Work out the finished part from the listing and answer in its coordinate system (mm). Face numbers are marked on the shaded views. A direction names the side the tool comes from. Coordinates: 2 decimals unless noted, no trailing zeros. Loops run counter-clockwise (first coordinate to the right, second up) from the corner with the lowest first, then second, coordinate; pieces in that order, holes last. Notation, with made-up numbers: (42.5, 66) -> (70.5, 66) arc R25 ccw to (70.5, 96) -> close; hole circle Ø6 at (34, 47.25). An arc over 180 degrees is marked (long way). One line per question, with ' | ' between items.
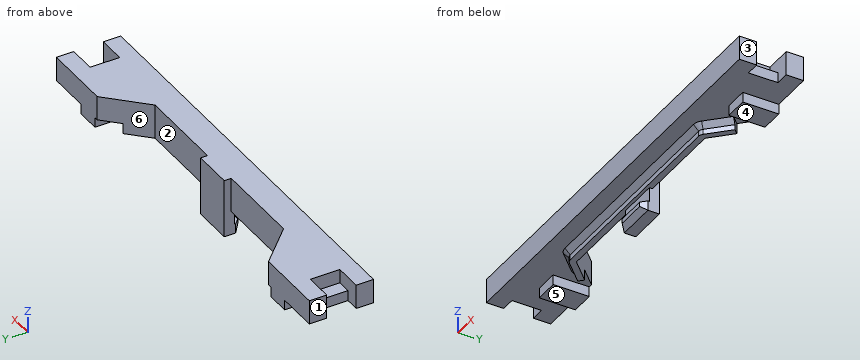
```python
from build123d import *

# Parameters (mm, degrees)
PAD002_DEPTH    = 7
PAD003_DEPTH    = 3
CHAMFER003_SIZE = 1.5
SKETCH019_W     = 4
SKETCH019_H     = 8.5
POCKET003_DEPTH = 7.001
SKETCH020_W     = 4
SKETCH020_H     = 8.5
POCKET004_DEPTH = 4
SKETCH024_W     = 11.6
SKETCH024_H     = 2.9
PAD006_DEPTH    = 16.9
SKETCH025_W     = 11.6
SKETCH025_H     = 2.8
PAD007_DEPTH    = 1.9
CHAMFER005_SIZE = 1.5
SKETCH026_W     = 6.8
SKETCH026_H     = 10.4
PAD008_DEPTH    = 2.9


with BuildPart() as part:
    # Sketch006 → Pad002 (new body)
    with BuildSketch(Plane.XY.offset(4)):
        Polygon((-62, 2.5), (-62, -16), (62, -16), (62, 2.5), (42, 2.5), (31.5, -8), (-31.5, -8), (-42, 2.5), align=None)
    extrude(amount=PAD002_DEPTH)

    # Sketch007 (on Face9 of Pad002) → Pad003 (join)
    with BuildSketch(Plane(origin=(0, 0, 4), x_dir=(1, 0, 0), z_dir=(0, 0, -1))):
        with BuildLine():
            Line((-31.5, 8), (31.5, 8))
            Line((37.293259, 2.206741), (31.5, 8))
            Line((38.566051, 3.479533), (37.293259, 2.206741))
            Line((32.772792, 9.272792), (38.566051, 3.479533))
            ThreePointArc((32.772792, 9.272792), (32.18883, 9.662983), (31.5, 9.8))
            Line((31.5, 9.8), (-31.5, 9.8))
            ThreePointArc((-31.5, 9.8), (-32.18883, 9.662983), (-32.772792, 9.272792))
            Line((-38.566051, 3.479533), (-32.772792, 9.272792))
            Line((-37.293259, 2.206741), (-38.566051, 3.479533))
            Line((-31.5, 8), (-37.293259, 2.206741))
        make_face()
    extrude(amount=PAD003_DEPTH)

    # Chamfer003
    chamfer003_edges = [part.edges().sort_by_distance(p)[0] for p in [
        (-35.669422, -6.376163, 4),
    ]]
    chamfer(chamfer003_edges, length=CHAMFER003_SIZE)

    # Sketch019 (on Face1 of Chamfer003) → Pocket003 (cut, through all)
    with BuildSketch(Plane(origin=(0, 0, 4), x_dir=(1, 0, 0), z_dir=(0, 0, -1))):
        with Locations((-60, 6.75)):
            Rectangle(SKETCH019_W, SKETCH019_H)
        with Locations((60, 6.75)):
            Rectangle(SKETCH019_W, SKETCH019_H)
    extrude(amount=-POCKET003_DEPTH, mode=Mode.SUBTRACT)

    # Sketch020 (on Face31 of Pocket003) → Pocket004 (cut)
    with BuildSketch(Plane.XY.offset(11)):
        with Locations((-56, -6.75)):
            Rectangle(SKETCH020_W, SKETCH020_H)
        with Locations((56, -6.75)):
            Rectangle(SKETCH020_W, SKETCH020_H)
    extrude(amount=-POCKET004_DEPTH, mode=Mode.SUBTRACT)

    # Sketch024 (on Face27 of Pocket004) → Pad006 (join)
    with BuildSketch(Plane.XY.offset(11)):
        with Locations((0, -7.45)):
            Rectangle(SKETCH024_W, SKETCH024_H)
    extrude(amount=-PAD006_DEPTH)

    # Sketch025 (on Face37 of Pad006) → Pad007 (join)
    with BuildSketch(Plane.XZ.offset(8.9)):
        with Locations((0, -4.5)):
            Rectangle(SKETCH025_W, SKETCH025_H)
    extrude(amount=PAD007_DEPTH)

    # Chamfer005
    chamfer005_edges = [part.edges().sort_by_distance(p)[0] for p in [
        (0, -10.8, -5.9),
        (-5.8, -10.8, -4.5),
        (5.8, -10.8, -4.5),
    ]]
    chamfer(chamfer005_edges, length=CHAMFER005_SIZE)

    # Sketch026 (on Face37 of Chamfer005) → Pad008 (join)
    with BuildSketch(Plane(origin=(0, 0, 4), x_dir=(1, 0, 0), z_dir=(0, 0, -1))):
        with Locations((-46.5, 2.7)):
            Rectangle(SKETCH026_W, SKETCH026_H)
        with Locations((46.5, 2.7)):
            Rectangle(SKETCH026_W, SKETCH026_H)
    extrude(amount=PAD008_DEPTH)


solid = part.part
```
1) Flat-ended cylindrical pins translate along their axes: pin 1 (2 mm diameter, centred on x = -1.5, z = -0.5, fed in from -Y); pin 2 (4 mm diameter, centred on x = 46.5, y = -1, fed in from -Z); pin 3 (4 mm diameter, centred on x = 14, y = -5, fed in from -Z); pin 4 (0.9 mm diameter, centred on y = -8.5, z = 5.5, fed in from +X). Find the tip coordinate at first contact, or state that the pin passes through.
Check values:
pin 1: stops at y = -8.9 | pin 2: stops at z = 1.1 | pin 3: passes through | pin 4: stops at x = 58
2) Find the intervals of material crossed by line 1 along Y through (x, z) = (-55, 7.75); line 2 along X through (y, z) = (-1, 2.75); line 3 along X through (y, z) = (-2.75, 2), in increasing order.
Check values:
line 1: y = -16 to -11, -2.5 to 2.5 | line 2: x = -49.9 to -43.1, 43.1 to 49.9 | line 3: x = -49.9 to -43.1, -37.84 to -36.75, 36.75 to 37.84, 43.1 to 49.9
3) Find section D-D (x = -10.5). Write down the section's boundary in (y, z), plus the area to 3 significant figures.
Check values:
outline: (-16, 4) -> (-11.3, 4) -> (-9.8, 2.5) -> (-9.8, 1) -> (-8, 1) -> (-8, 11) -> (-16, 11) -> close | area: 62.5 mm^2
4) Find section C-C (z = -1.75). Write down the section's boundary in (x, y).
Check values:
outline: (-5.8, -8.9) -> (5.8, -8.9) -> (5.8, -6) -> (-5.8, -6) -> close
5) For the marked faces 4, 5 and 6, determine the directions among +Z, -Z, +X, -X, +Y, -Y from which every point of the face is accessible in a straight line to the end or side of a thin tool.
Check values:
face 4: -Z, +X, +Y, -Y | face 5: -Z, -X, +Y, -Y | face 6: +Z, -Z, +Y
6) Find section B-B (x = 2). Write down the section's boundary in (y, z).
Check values:
outline: (-16, 4) -> (-11.3, 4) -> (-9.8, 2.5) -> (-9.8, 1) -> (-8.9, 1) -> (-8.9, -3.1) -> (-10.8, -3.1) -> (-10.8, -4.4) -> (-9.3, -5.9) -> (-6, -5.9) -> (-6, 11) -> (-16, 11) -> close
7) The mould has two halves that part along X. Classify the marked faces 1, 2 and 3: released by +X, released by -X, zero draft, split by the parting line, or undercut.
Check values:
face 1: released by -X | face 2: undercut | face 3: released by +X
8) Find section A-A (y = -0.25). Write down the section's boundary in (x, z).
Check values:
outline: (-62, 4) -> (-49.9, 4) -> (-49.9, 1.1) -> (-43.1, 1.1) -> (-43.1, 4) -> (-39.25, 4) -> (-39.25, 11) -> (-62, 11) -> close; (39.25, 4) -> (43.1, 4) -> (43.1, 1.1) -> (49.9, 1.1) -> (49.9, 4) -> (62, 4) -> (62, 11) -> (39.25, 11) -> close
